```python
from build123d import *

# Parameters (mm, degrees)
F1_DEPTH = 25
F2_R     = 2
F4_COUNT = 9


with BuildPart() as f1:
    # F0 (on Front) → F1 (new body)
    with BuildSketch(Plane.XZ):
        with BuildLine():
            ThreePointArc((-6, 24.269322), (-15.411035, -19.68502), (25, 0))
            ThreePointArc((25, 0), (19.68502, 15.411035), (6, 24.269322))
            ThreePointArc((6, 24.269322), (0, 25), (-6, 24.269322))
        make_face()
        with BuildLine():
            ThreePointArc((-6, 24.269322), (0, 25), (6, 24.269322))
            Line((6, 24.269322), (6, 28))
            ThreePointArc((6, 28), (5.154701, 29.632993), (3.333333, 29.885618))
            ThreePointArc((3.333333, 29.885618), (0, 29.313708), (-3.333333, 29.885618))
            ThreePointArc((-3.333333, 29.885618), (-5.154701, 29.632993), (-6, 28))
            Line((-6, 28), (-6, 24.269322))
        make_face()
    extrude(amount=F1_DEPTH)

    # F2
    f2_edges = [f1.edges().sort_by_distance(p)[0] for p in [
        (-6, -12.5, 24.269322),
        (6, -12.5, 24.269322),
    ]]
    fillet(f2_edges, radius=F2_R)

    # F4: F1 ×9 about axis
    f4_axis = Axis((0, -14.063225, 0), (0, -1, 0))


with BuildPart() as f1_1:
    add(f1.part)
    for i in range(1, F4_COUNT):
        add(f1.part.rotate(f4_axis, i * 360 / F4_COUNT))


solid = f1_1.part
```
Build history of the part. All positions in model axes, mm. A direction names the side the tool comes from. Give positions to 0.01 mm unless a question says otherwise; leave off trailing zeros. Loops run counter-clockwise (first coordinate to the right, second up) from the corner with the lowest first, then second, coordinate; pieces in that order, holes last.
Item 1: Drill centre lines: line 1 (X direction, y = -16.5, z = 24); line 2 (X direction, y = -19.5, z = 27); line 3 (X direction, y = -2.5, z = 7). Where is each one in solid material? Low to high.
Answers follow:
line 1: x = -17.36 to -12.31, -7.1 to 7.1, 12.31 to 17.36
line 2: x = -6 to 6
line 3: x = -28.72 to 28.72
Item 2: Flat gauge pins, fed straight in: pin 1 (0.7 mm diameter, centred on y = -16.5, z = 26.5, fed in from -X); pin 2 (8 mm diameter, centred on y = -6.5, z = 12, fed in from +X); pin 3 (10 mm diameter, centred on x = -3.5, z = 14, fed in from +Y); pin 4 (8 mm diameter, centred on x = 17.5, y = -19.5, fed in from +Z). Where does each tip first touch, or does it go through?
Answers follow:
pin 1: stops at x = -6
pin 2: stops at x = 28.88
pin 3: stops at y = 0
pin 4: stops at z = 26.02
Item 3: Which spindle directions (+Z, -Z, +X, -X, +Y, -Y) get a long thin tool onto all of the face, cutting with end or side? Do faces 5 (the face through (21.659, -12.325, 12.485)), 6 (the face through (8.566, -12.325, 23.487)), 7 (the face through (3.555, -12.325, -27.309)), 8 (the face through (-25.41, -12.32, -14.62)). Say none if no direction does.
Answers follow:
face 5: +X, +Y, -Y
face 6: +Z, +Y, -Y
face 7: -Z, +Y, -Y
face 8: -Z, -X, +Y, -Y
Item 4: Slice it at A-A, the plane z = -17. List the corners of the cut face in (x, y).
Answers follow:
outline: (-24.41, -25) - (24.41, -25) - (24.41, 0) - (-24.41, 0) - close
Item 5: Pull direction X, two halves, no side cores. Call faces 1 (the face through (-14.424, -12.675, -20.915)), 2 (the face through (-8.53, -12.32, 23.5)), 3 (the face through (-15.072, -12.325, 26.016)), 4 (the face through (23.003, -12.325, 19.361)): released by +X, released by -X, zero draft, split by the parting line, or undercut.
Answers follow:
face 1: released by -X
face 2: undercut
face 3: undercut
face 4: released by +X
